Build history of the part. All positions in model axes, mm. A direction names the side the tool comes from. Give positions to 0.01 mm unless a question says otherwise; leave off trailing zeros. Order: outer loops, then holes, each group sorted by start corner. A loop starts at its lowest first (then second) coordinate and runs counter-clockwise, first axis right, second up. Notation, with made-up numbers: (64.25, 89) -> (69.25, 89) arc R9 cw to (69.25, 103) -> close; hole circle Ø1 at (85.25, -22.75). An arc over 180 degrees is marked (long way). Use a Markdown table: item, result. Add a question column.
```python
from build123d import *

# Parameters (mm, degrees)
SKETCH2_W               = 200
SKETCH2_H               = 200
BOSS_EXTRUDE1_DEPTH     = 70
SHELL2_T                = -2
CUT_EXTRUDE1_DEPTH      = 1
CUT_EXTRUDE1_DEPTH_BACK = 201
SKETCH5_W               = 22
SKETCH5_H               = 26
CUT_EXTRUDE2_DEPTH      = 7
SKETCH6_W               = 27
SKETCH6_H               = 19
CUT_EXTRUDE3_DEPTH      = 7
SKETCH7_R               = 2.5
CUT_EXTRUDE4_DEPTH      = 7
SKETCH8_R               = 5
CUT_EXTRUDE5_DEPTH      = 2
FILLET2_R               = 2


with BuildPart() as part:
    # Sketch2 → Boss-Extrude1 (new body)
    with BuildSketch(Plane(origin=(0, 0, 0), x_dir=(1, 0, 0), z_dir=(0, 1, 0))):
        with Locations((-100, -100)):
            Rectangle(SKETCH2_W, SKETCH2_H)
    extrude(amount=BOSS_EXTRUDE1_DEPTH)

    # Shell2
    shell2_openings = [part.faces().sort_by_distance(p)[0] for p in [
        (-100, 70, 100),
    ]]
    offset(amount=SHELL2_T, openings=shell2_openings, kind=Kind.INTERSECTION)

    # Sketch3 → Cut-Extrude1 (cut, two sides)
    with BuildSketch(Plane.XY.offset(200)) as cut_extrude1_sk:
        with BuildLine():
            Line((-180, 65), (-20, 65))
            ThreePointArc((-20, 65), (-17.5, 62.5), (-20, 60))
            Line((-20, 60), (-180, 60))
            ThreePointArc((-180, 60), (-182.5, 62.5), (-180, 65))
        make_face()
        with BuildLine():
            Line((-180, 55), (-20, 55))
            ThreePointArc((-20, 55), (-17.5, 52.5), (-20, 50))
            Line((-20, 50), (-180, 50))
            ThreePointArc((-180, 50), (-182.5, 52.5), (-180, 55))
        make_face()
        with BuildLine():
            Line((-180, 45), (-20, 45))
            ThreePointArc((-20, 45), (-17.5, 42.5), (-20, 40))
            Line((-20, 40), (-180, 40))
            ThreePointArc((-180, 40), (-182.5, 42.5), (-180, 45))
        make_face()
        with BuildLine():
            Line((-180, 35), (-20, 35))
            ThreePointArc((-20, 35), (-17.5, 32.5), (-20, 30))
            Line((-20, 30), (-180, 30))
            ThreePointArc((-180, 30), (-182.5, 32.5), (-180, 35))
        make_face()
    extrude(amount=CUT_EXTRUDE1_DEPTH, mode=Mode.SUBTRACT)
    extrude(cut_extrude1_sk.sketch, amount=-CUT_EXTRUDE1_DEPTH_BACK, mode=Mode.SUBTRACT)

    # Sketch5 → Cut-Extrude2 (cut)
    with BuildSketch(Plane(origin=(0, 0, 0), x_dir=(0, 0, -1), z_dir=(1, 0, 0))):
        with Locations((-21, 23)):
            Rectangle(SKETCH5_W, SKETCH5_H)
    extrude(amount=-CUT_EXTRUDE2_DEPTH, mode=Mode.SUBTRACT)

    # Sketch6 → Cut-Extrude3 (cut)
    with BuildSketch(Plane.ZY.offset(200)):
        with Locations((171.5, 19.5)):
            Rectangle(SKETCH6_W, SKETCH6_H)
    extrude(amount=-CUT_EXTRUDE3_DEPTH, mode=Mode.SUBTRACT)

    # Sketch7 → Cut-Extrude4 (cut)
    with BuildSketch(Plane(origin=(0, 0, 0), x_dir=(0, 0, -1), z_dir=(1, 0, 0))):
        with Locations((-180, 20)):
            Circle(SKETCH7_R)
        with Locations((-165, 20)):
            Circle(SKETCH7_R)
    extrude(amount=-CUT_EXTRUDE4_DEPTH, mode=Mode.SUBTRACT)

    # Sketch8 → Cut-Extrude5 (cut)
    with BuildSketch(Plane(origin=(0, 0, 0), x_dir=(0, 0, -1), z_dir=(1, 0, 0))):
        with Locations((-10, 60)):
            Circle(SKETCH8_R)
    extrude(amount=-CUT_EXTRUDE5_DEPTH, mode=Mode.SUBTRACT)

    # Fillet2
    fillet2_edges = [part.edges().sort_by_distance(p)[0] for p in [
        (0, 35, 200),
        (-200, 35, 200),
        (-200, 35, 0),
        (0, 35, 0),
    ]]
    fillet(fillet2_edges, radius=FILLET2_R)


solid = part.part
```
(1) Mould opens along Z. For faces 4 (the face through (0, 35, 101)), 5 (the face through (-101, 27, 0)), 6 (the face through (-2, 36, 101)) say: released by +Z, released by -Z, zero draft, split by the parting line, or undercut.
(2) Band-saw the part on D-D on z = 180. Give the cut face in (x, y), plus the area to 3 significant figures.
(3) Band-saw the part on A-A on y = 32.5. Give the cut face in (x, z), plus the area to 3 significant figures.
(4) Band-saw the part on B-B on z = 29. Give the cut face in (x, y).
(5) Wall check: probe 1 along Y at (x, z) = (-1, 180); probe 2 along X at (y, z) = (10, 157); probe 3 along Z at (x, y) = (-151.5, 11.5). Give the ranges that are in metal, low to high.
(6) Band-saw the part on C-C on x = -187. Give the cut face in (y, z), plus the area to 3 significant figures.
(7) Tool access for faces 1 (the face through (-1, 64, 7)), 2 (the face through (-101, 36, 198)), 3 (the face through (-101, 0, 99)): list every direction of +Z, -Z, +X, -X, +Y, -Y with a clear straight run to the whole face (end or side of a thin tool).
(8) Pin check, flat tips, straight feed: pin 1 Ø1.6 at (x, y) = (-1, 23) entering from +Z; pin 2 Ø5 at (x, z) = (-166, 107) entering from +Y. Stop position of each tip, or through.
Response:
| question | item | result |
|---|---|---|
| 1 | face 4 | zero draft |
| 1 | face 5 | released by -Z |
| 1 | face 6 | undercut |
| 2 | outline | (-200, 0) -> (0, 0) -> (0, 17.5) -> (-2, 17.5) -> (-2, 2) -> (-198, 2) -> (-198, 10) -> (-200, 10) -> close; (-200, 29) -> (-198, 29) -> (-198, 70) -> (-200, 70) -> close; (-2, 22.5) -> (0, 22.5) -> (0, 70) -> (-2, 70) -> close |
| 2 | area | 624 mm² |
| 3 | outline | (-200, 2) arc R2 ccw to (-198, 0) -> (-182.5, 0) -> (-182.5, 2) -> (-198, 2) -> (-198, 198) -> (-182.5, 198) -> (-182.5, 200) -> (-198, 200) arc R2 ccw to (-200, 198) -> close; (-17.5, 0) -> (-2, 0) arc R2 ccw to (0, 2) -> (0, 10) -> (-2, 10) -> (-2, 2) -> (-17.5, 2) -> close; (-17.5, 198) -> (-2, 198) -> (-2, 32) -> (0, 32) -> (0, 198) arc R2 ccw to (-2, 200) -> (-17.5, 200) -> close |
| 3 | area | 877 mm² |
| 4 | outline | (-200, 0) -> (0, 0) -> (0, 10) -> (-2, 10) -> (-2, 2) -> (-198, 2) -> (-198, 70) -> (-200, 70) -> close; (-2, 36) -> (0, 36) -> (0, 70) -> (-2, 70) -> close |
| 5 | probe 1 | y = 0 to 17.5, 22.5 to 70 |
| 5 | probe 2 | x = -200 to -198, -2 to 0 |
| 5 | probe 3 | z = 0 to 2, 198 to 200 |
| 6 | outline | (0, 0) -> (70, 0) -> (70, 2) -> (2, 2) -> (2, 198) -> (70, 198) -> (70, 200) -> (0, 200) -> close |
| 6 | area | 672 mm² |
| 7 | face 1 | +X |
| 7 | face 2 | +Y |
| 7 | face 3 | +Z, -Z, +X, -X, -Y |
| 8 | pin 1 | stops at z = 199.99 |
| 8 | pin 2 | stops at y = 2 |
